from build123d import *

# Parameters (mm, degrees)
BOSS_EXTRUDE1_DEPTH = 10


with BuildPart() as part:
    # Sketch1 → Boss-Extrude1 (new body)
    with BuildSketch(Plane.XY):
        with BuildLine():
            Line((-20.5, -6), (-15.5, -6))
            ThreePointArc((-15.5, -6), (-14.095, -7.405), (-15.5, -8.81))
            Line((-15.5, -8.81), (-20.5, -8.81))
            ThreePointArc((-20.5, -8.81), (-22.486970055, -7.986970055), (-23.31, -6))
            Line((-23.31, -6), (-23.31, 6))
            ThreePointArc((-23.31, 6), (-22.486970055, 7.986970055), (-20.5, 8.81))
            Line((-20.5, 8.81), (-8.31, 8.81))
            Line((-8.31, 8.81), (-8.31, 9.5))
            ThreePointArc((-8.31, 9.5), (-7.486970055, 11.486970055), (-5.5, 12.31))
            Line((-5.5, 12.31), (5.5, 12.31))
            ThreePointArc((5.5, 12.31), (7.486970055, 11.486970055), (8.31, 9.5))
            Line((8.31, 9.5), (8.31, 8.81))
            Line((8.31, 8.81), (20.5, 8.81))
            ThreePointArc((20.5, 8.81), (22.486970055, 7.986970055), (23.31, 6))
            Line((23.31, 6), (23.31, -6))
            ThreePointArc((23.31, -6), (22.486970055, -7.986970055), (20.5, -8.81))
            Line((20.5, -8.81), (15.5, -8.81))
            ThreePointArc((15.5, -8.81), (14.095, -7.405), (15.5, -6))
            Line((15.5, -6), (20.5, -6))
            Line((20.5, -6), (20.5, 6))
            Line((20.5, 6), (8.31, 6))
            ThreePointArc((8.31, 6), (6.323029945, 6.823029945), (5.5, 8.81))
            Line((5.5, 8.81), (5.5, 9.5))
            Line((5.5, 9.5), (-5.5, 9.5))
            Line((-5.5, 9.5), (-5.5, 8.81))
            ThreePointArc((-5.5, 8.81), (-6.323029945, 6.823029945), (-8.31, 6))
            Line((-8.31, 6), (-20.5, 6))
            Line((-20.5, 6), (-20.5, -6))
        make_face()
    extrude(amount=BOSS_EXTRUDE1_DEPTH)


solid = part.part
Check sheet for the modelled part. Datum: model origin and axes. Units: mm. A direction names the side the tool comes from. Give positions to 0.01 mm unless a question says otherwise; leave off trailing zeros. Order: outer loops, then holes, each group sorted by start corner. A loop starts at its lowest first (then second) coordinate and runs counter-clockwise, first axis right, second up. Notation, with made-up numbers: (10, 27) - (47, 27) arc R8 cw to (47, 34) - close; hole circle Ø7 at (60, 47.25). An arc over 180 degrees is marked (long way). Answer as CSV lines item,"result".
1. Section check C-C (y = 7). Record the boundary of the cut face in (x, z).
Result sheet:
outline,"(-23.13, 0) - (-6.16, 0) - (-6.16, 10) - (-23.13, 10) - close; (6.16, 0) - (23.13, 0) - (23.13, 10) - (6.16, 10) - close"
2. Section check B-B (z = 9.5). Record the boundary of the cut face in (x, y) (3 decimals), then the cut area to 3 significant figures.
Result sheet:
outline,"(-23.31, -6) arc R2.81 ccw to (-20.5, -8.81) - (-15.5, -8.81) arc R1.405 ccw to (-15.5, -6) - (-20.5, -6) - (-20.5, 6) - (-8.31, 6) arc R2.81 ccw to (-5.5, 8.81) - (-5.5, 9.5) - (5.5, 9.5) - (5.5, 8.81) arc R2.81 ccw to (8.31, 6) - (20.5, 6) - (20.5, -6) - (15.5, -6) arc R1.405 ccw to (15.5, -8.81) - (20.5, -8.81) arc R2.81 ccw to (23.31, -6) - (23.31, 6) arc R2.81 ccw to (20.5, 8.81) - (8.31, 8.81) - (8.31, 9.5) arc R2.81 ccw to (5.5, 12.31) - (-5.5, 12.31) arc R2.81 ccw to (-8.31, 9.5) - (-8.31, 8.81) - (-20.5, 8.81) arc R2.81 ccw to (-23.31, 6) - close"
area,"255 mm²"
3. Go/stop test with flat-tipped pins: P1, Ø6, axis at x = -10.5, z = 7.5, coming from the -Y side; P2, Ø2, axis at x = -7.5, z = 4.5, coming from the +Y side; P3, Ø5.5, axis at x = 18.5, z = 3, coming from the +Y side. Record where each tip stops, or that it passes through.
Result sheet:
P1,"y = 6"
P2,"y = 12.13"
P3,"y = 8.81"
4. Section check A-A (y = -1.75). Record the boundary of the cut face in (x, z), then the cut area to 3 significant figures.
Result sheet:
outline,"(-23.31, 0) - (-20.5, 0) - (-20.5, 10) - (-23.31, 10) - close; (20.5, 0) - (23.31, 0) - (23.31, 10) - (20.5, 10) - close"
area,"56.2 mm²"
5. Scan lines: probe 1 along X at (y, z) = (5.5, 0.75); probe 2 along Y at (x, z) = (-17.5, 9); probe 3 along X at (y, z) = (8, 8). Record each from-to range of solid material in increasing order. Write a range as from..to.
Result sheet:
probe 1,"-23.31..-20.5, 20.5..23.31"
probe 2,"-8.81..-6, 6..8.81"
probe 3,"-22.47..-5.62, 5.62..22.47"
6. Tool access check on faces 5 (the face through (18, -8.81, 5)), 6 (the face through (-14.095, -7.374, 4.93)), 7 (the face through (0, 9.5, 5)). Record the directions out of +Z, -Z, +X, -X, +Y, -Y that give a thin tool (end or side, any length) a straight path to the whole face; none if there is none.
Result sheet:
face 5,"+Z, -Z, +X, -X, -Y"
face 6,"+Z, -Z"
face 7,"+Z, -Z, -Y"
7. Mould release check, pull along Y, two halves, no side actions. Record for faces 1 (the face through (-6.301, 6.845, 4.93)), 2 (the face through (-14, 6, 5)), 3 (the face through (23.31, 0, 5)), 4 (the face through (7.465, 11.509, 4.93)): released by +Y, released by -Y, zero draft, split by the parting line, or undercut.
Result sheet:
face 1,"released by -Y"
face 2,"undercut"
face 3,"zero draft"
face 4,"released by +Y"
8. Section check D-D (x = -11). Record the boundary of the cut face in (y, z), then the cut area to 3 significant figures.
Result sheet:
outline,"(6, 0) - (8.81, 0) - (8.81, 10) - (6, 10) - close"
area,"28.1 mm²"
